The model under review builds one solid part; all positions refer to its coordinate system, in mm. Face numbers are marked on the shaded views. A direction names the side the tool comes from. Round coordinates to 2 decimals unless told otherwise and drop trailing zeros. Write each loop counter-clockwise with the first axis right and the second up, starting at its lowest first coordinate (ties: lowest second). Pieces come first, ordered by that corner, then holes. Notation, with made-up numbers: (-29.5, 85.25) -> (-3.5, 85.25) arc R5 ccw to (-3.5, 91.25) -> close; hole circle Ø7 at (-6.5, -6). An arc over 180 degrees is marked (long way). Answer in a Markdown table with one row per item. Add a question column.
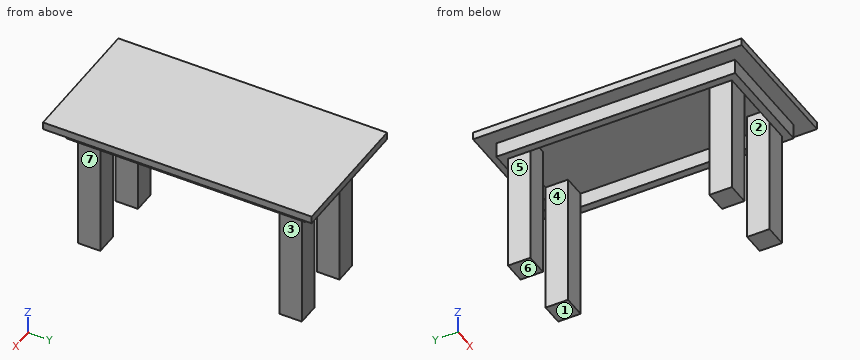
```python
from build123d import *

# Parameters (mm, degrees)
F0_W     = 914.4
F0_H     = 1828.8
F1_DEPTH = 50.8
F2_W     = 711.2
F2_H     = 1625.6
F2_W_2   = 609.6
F2_H_2   = 1524
F3_DEPTH = 101.6
F5_W     = 152.4
F5_H     = 152.4
F4_DEPTH = 914.4


with BuildPart() as f1:
    # F0 (on Top) → F1 (new body)
    with BuildSketch(Plane.XY):
        Rectangle(F0_W, F0_H)
    extrude(amount=-F1_DEPTH)

    # F2 (on face) → F3 (join)
    with BuildSketch(Plane(origin=(0, 0, -50.8), x_dir=(1, 0, 0), z_dir=(0, 0, -1))):
        Rectangle(F2_W, F2_H)
        Rectangle(F2_W_2, F2_H_2, mode=Mode.SUBTRACT)
    extrude(amount=F3_DEPTH)

    # F5 (on face) → F4 (join)
    with BuildSketch(Plane(origin=(0, 0, -50.8), x_dir=(1, 0, 0), z_dir=(0, 0, -1))):
        with Locations((-228.6, -685.8)):
            Rectangle(F5_W, F5_H)
        with Locations((-228.6, 685.8)):
            Rectangle(F5_W, F5_H)
        with Locations((228.6, -685.8)):
            Rectangle(F5_W, F5_H)
        with Locations((228.6, 685.8)):
            Rectangle(F5_W, F5_H)
    extrude(amount=F4_DEPTH)


solid = f1.part
```
1. Add section B-B on z = -85. Write out the cut boundary in (x, y).
2. For L1, parallel to Y at x = -241, z = -796; L2, parallel to X at y = -703, z = -500; L3, parallel to Y at x = -10.5, z = -96, list the stretches that pass through material, from the lowest coordinate up.
3. Add section A-A on z = -447.5. Write out the cut boundary in (x, y).
4. Add section C-C on y = -110. Write out the cut boundary in (x, z).
5. Insertion check: pin 1 Ø8 at (x, z) = (-243, -135) entering from +Y; pin 2 Ø3 at (x, y) = (271.5, -548) entering from +Z; pin 3 Ø10 at (x, y) = (337, 423.5) entering from -Z; pin 4 Ø1.5 at (x, z) = (-238.5, -616.5) entering from -Y. Each pin has a flat end and moves straight along its axis. Give the tip position at first contact, or say it passes through.
6. Tool access review of the marked faces 5, 6 and 7: name each direction out of +Z, -Z, +X, -X, +Y, -Y from which nothing blocks a thin tool from reaching the whole face with its end or side.
7. Add section D-D on x = -26. Write out the cut boundary in (y, z).
8. Mouldability with a two-part tool opening along X and no side actions: class the marked faces 1, 2, 3 and 4 as pulls with the +X half, pulls with the -X half, needs draft (parallel to the pull), parting line crosses it, or undercut.
Filled in:
| question | item | result |
|---|---|---|
| 1 | outline | (-355.6, -812.8) -> (355.6, -812.8) -> (355.6, 812.8) -> (-355.6, 812.8) -> close; hole (-304.8, -609.6) -> (-152.4, -609.6) -> (-152.4, -762) -> (152.4, -762) -> (152.4, -609.6) -> (304.8, -609.6) -> (304.8, 609.6) -> (152.4, 609.6) -> (152.4, 762) -> (-152.4, 762) -> (-152.4, 609.6) -> (-304.8, 609.6) -> close |
| 2 | L1 | -762 to -609.6, 609.6 to 762 |
| 2 | L2 | -304.8 to -152.4, 152.4 to 304.8 |
| 2 | L3 | -812.8 to -762, 762 to 812.8 |
| 3 | outline | (-304.8, -762) -> (-152.4, -762) -> (-152.4, -609.6) -> (-304.8, -609.6) -> close; (-304.8, 609.6) -> (-152.4, 609.6) -> (-152.4, 762) -> (-304.8, 762) -> close; (152.4, -762) -> (304.8, -762) -> (304.8, -609.6) -> (152.4, -609.6) -> close; (152.4, 609.6) -> (304.8, 609.6) -> (304.8, 762) -> (152.4, 762) -> close |
| 4 | outline | (-457.2, -50.8) -> (-355.6, -50.8) -> (-355.6, -152.4) -> (-304.8, -152.4) -> (-304.8, -50.8) -> (304.8, -50.8) -> (304.8, -152.4) -> (355.6, -152.4) -> (355.6, -50.8) -> (457.2, -50.8) -> (457.2, 0) -> (-457.2, 0) -> close |
| 5 | pin 1 | y = 812.8 |
| 5 | pin 2 | z = 0 |
| 5 | pin 3 | z = -152.4 |
| 5 | pin 4 | y = -762 |
| 6 | face 5 | -Z, -X, +Y, -Y |
| 6 | face 6 | -Z, +X, -X, +Y, -Y |
| 6 | face 7 | -Z, +X, +Y, -Y |
| 7 | outline | (-914.4, -50.8) -> (-812.8, -50.8) -> (-812.8, -152.4) -> (-762, -152.4) -> (-762, -50.8) -> (762, -50.8) -> (762, -152.4) -> (812.8, -152.4) -> (812.8, -50.8) -> (914.4, -50.8) -> (914.4, 0) -> (-914.4, 0) -> close |
| 8 | face 1 | needs draft |
| 8 | face 2 | undercut |
| 8 | face 3 | pulls with the +X half |
| 8 | face 4 | undercut |
